```python
from build123d import *

# Parameters (mm, degrees)
SKETCH_1_R      = 1.35
EXTRUDE_1_DEPTH = 3


with BuildPart() as part:
    # 草图1 → 凸台-拉伸1 (new body)
    with BuildSketch(Plane.XY.offset(3)):
        with BuildLine():
            Line((-6.157118156, 20.9998), (-6.157118156, 3))
            ThreePointArc((-6.157118156, 3), (-5.2784385, 0.878679656), (-3.157118156, 0))
            Line((-3.157118156, 0), (13.843681844, 0))
            Line((13.843681844, 0), (24.001386189, 0.533010723))
            ThreePointArc((24.001386189, 0.533010723), (26.020372671, 1.463896655), (26.844181844, 3.528889024))
            Line((26.844181844, 3.528889024), (26.844181844, 20.471910982))
            ThreePointArc((26.844181844, 20.471910982), (26.020271299, 22.537010177), (24.001092054, 23.467804703))
            Line((24.001092054, 23.467804703), (13.843681844, 23.9998))
            Line((13.843681844, 23.9998), (-3.157118156, 23.9998))
            ThreePointArc((-3.157118156, 23.9998), (-5.2784385, 23.121120344), (-6.157118156, 20.9998))
        make_face()
        with Locations(Location((-3.156018156, 20.498351651, 0), (0, 0, 180))):
            Circle(SKETCH_1_R, mode=Mode.SUBTRACT)
        with Locations(Location((24.044031844, 20.498351651, 0), (0, 0, 180))):
            Circle(SKETCH_1_R, mode=Mode.SUBTRACT)
        with Locations(Location((-3.156018156, 3.501148349, 0), (0, 0, 180))):
            Circle(SKETCH_1_R, mode=Mode.SUBTRACT)
        with Locations(Location((24.044031844, 3.501148349, 0), (0, 0, 180))):
            Circle(SKETCH_1_R, mode=Mode.SUBTRACT)
        Polygon((23.343481844, 9.5), (21.843181844, 9.5), (21.843181844, 6), (16.343381844, 6), (16.343381844, 3), (4.343381844, 3), (4.343381844, 6), (-1.156518156, 6), (-1.156518156, 9.5), (-2.656818156, 9.5), (-2.656818156, 14.4995), (-1.156518156, 14.4995), (-1.156518156, 17.9998), (4.343381844, 17.9998), (4.343381844, 20.9998), (16.343381844, 20.9998), (16.343381844, 17.9998), (21.843181844, 17.9998), (21.843181844, 14.4995), (23.343481844, 14.4995), align=None, mode=Mode.SUBTRACT)
    extrude(amount=-EXTRUDE_1_DEPTH)


solid = part.part
```
Work out the finished part from the listing and answer in its coordinate system (mm). A direction names the side the tool comes from. Give positions to 0.01 mm unless a question says otherwise; leave off trailing zeros. Write each loop counter-clockwise with the first axis right and the second up, starting at its lowest first coordinate (ties: lowest second). Pieces come first, ordered by that corner, then holes.
(1) Flat-ended cylindrical pins translate along their axes: pin 1 Ø8 at (x, y) = (10.5, 15) entering from -Z; pin 2 Ø2 at (x, y) = (5.5, 20.5) entering from +Z; pin 3 Ø0.9 at (x, z) = (19, 2) entering from -Y; pin 4 Ø0.8 at (x, z) = (22.5, 1.5) entering from -Y. Find the tip coordinate at first contact, or state that the pin passes through.
Final values:
pin 1: passes through
pin 2: stops at z = 3
pin 3: stops at y = 0.25
pin 4: stops at y = 0.43
(2) Which of the six approach directions +Z, -Z, +X, -X, +Y, -Y give full straight-line access (tool end or side, diameter ignored) to faces 4 (the flat face through (10, 21, 2)), 5 (the flat face through (5, 0, 2))?
Final values:
face 4: +Z, -Z
face 5: +Z, -Z, +X, -X, -Y
(3) The mould has two halves that part along Y. Classify faces 1 (the cylindrical face through (25.115, 4.323, 1.521)), 2 (the flat face through (18.851, 0.263, 1.521)), 3 (the flat face through (18.99, 23.73, 1.52)): pulls with the +Y half, pulls with the -Y half, needs draft (parallel to the pull), parting line crosses it, or undercut.
Final values:
face 1: undercut
face 2: pulls with the -Y half
face 3: pulls with the +Y half
(4) The part is cut by section C-C on z = 1.6. Count the separate pieces of the cut face and the enclosed holes in it, plus the area to 3 significant figures.
Final values:
separate pieces: 1
enclosed holes: 5
area: 390 mm2
(5) The part is cut by section D-D on x = 25. Write down the section's boundary in (y, z), plus the area to 3 significant figures.
Final values:
outline: (0.76, 0) - (2.55, 0) - (2.55, 3) - (0.76, 3) - close; (4.45, 0) - (19.55, 0) - (19.55, 3) - (4.45, 3) - close; (21.45, 0) - (23.24, 0) - (23.24, 3) - (21.45, 3) - close
area: 56.0 mm2
(6) The part is cut by section A-A on x = 1. Write down the section's boundary in (y, z).
Final values:
outline: (0, 0) - (6, 0) - (6, 3) - (0, 3) - close; (18, 0) - (24, 0) - (24, 3) - (18, 3) - close
(7) The part is cut by section B-B on y = 15. Write down the section's boundary in (x, z).
Final values:
outline: (-6.16, 0) - (-1.16, 0) - (-1.16, 3) - (-6.16, 3) - close; (21.84, 0) - (26.84, 0) - (26.84, 3) - (21.84, 3) - close
(8) Straight lines are drawn through the part: line 1 (Y direction, x = 11, z = 2.6); line 2 (Y direction, x = 2.5, z = 2.45); line 3 (X direction, y = 7, z = 0.85). For each, find the intervals that lie inside material, in ascending order.
Final values:
line 1: y = 0 to 3, 21 to 24
line 2: y = 0 to 6, 18 to 24
line 3: x = -6.16 to -1.16, 21.84 to 26.84
